from build123d import *

# Parameters (mm, degrees)
SKETCH1_W           = 241.3
SKETCH1_H           = 44.45
BOSS_EXTRUDE1_DEPTH = 19.06
SKETCH3_R           = 4
CUT_EXTRUDE1_DEPTH  = 125.151748779
CUT_EXTRUDE2_DEPTH  = 125.151748779
SKETCH11_R          = 15.113
CUT_EXTRUDE3_DEPTH  = 125.151748779
CUT_EXTRUDE5_DEPTH  = 125.151748779
FILLET1_R           = 3.175


with BuildPart() as part:
    # Sketch1 → Boss-Extrude1 (new body)
    with BuildSketch(Plane.XY):
        Rectangle(SKETCH1_W, SKETCH1_H)
    extrude(amount=BOSS_EXTRUDE1_DEPTH)

    # Sketch3 → Cut-Extrude1 (cut, through all)
    with BuildSketch(Plane.XY.offset(19.06)):
        with Locations((-107.95, 0)):
            Circle(SKETCH3_R)
    extrude(amount=-CUT_EXTRUDE1_DEPTH, mode=Mode.SUBTRACT)

    # Sketch5 → Cut-Extrude2 (cut, through all)
    with BuildSketch(Plane.XY.offset(19.06)):
        with BuildLine():
            ThreePointArc((67.637087091, -22.225), (96.497916739, -2.807923084), (120.65, 22.225))
            Line((120.65, 22.225), (120.65, -22.225))
            Line((120.65, -22.225), (67.637087091, -22.225))
        make_face()
        with BuildLine():
            Line((-61.710210997, -22.225), (-110.410681995, -9.201666649))
            ThreePointArc((-110.410681995, -9.201666649), (-117.466687359, 0.397852617), (-109.634072253, 9.374941368))
            Line((-109.634072253, 9.374941368), (-38.1, 22.225))
            Line((-38.1, 22.225), (-120.65, 22.225))
            Line((-120.65, 22.225), (-120.65, -22.225))
            Line((-120.65, -22.225), (-61.710210997, -22.225))
        make_face()
    extrude(amount=-CUT_EXTRUDE2_DEPTH, mode=Mode.SUBTRACT)

    # Sketch11 → Cut-Extrude3 (cut, through all)
    with BuildSketch(Plane(origin=(0, 0, 0), x_dir=(-1, 0, 0), z_dir=(0, 0, -1))):
        with Locations((-57.15, 0)):
            Circle(SKETCH11_R)
    extrude(amount=-CUT_EXTRUDE3_DEPTH, mode=Mode.SUBTRACT)

    # Sketch14 → Cut-Extrude5 (cut, through all)
    with BuildSketch(Plane.XY.offset(19.06)):
        Polygon((87.427282936, 15.558708401), (94.741989073, 6.41532573), (108.43714596, 17.350301349), align=None)
        Polygon((18.258483502, 14.338005817), (29.973493873, -13.800738505), (-32.606529101, -13.800738505), align=None)
        Polygon((-43.100879601, -13.800738505), (3.468328331, 11.961548148), (-56.519992491, 10.456326363), align=None)
        Polygon((-64.730780564, 8.662121496), (-52.068091334, -13.800738505), (-97.910045601, -2.558530136), align=None)
        Polygon((25.377220315, 10.456326363), (27.958556135, 4.256114298), (42.851089432, 10.456326363), align=None)
    extrude(amount=-CUT_EXTRUDE5_DEPTH, mode=Mode.SUBTRACT)

    # Fillet1
    # the kernel refuses this fillet: 3.175 mm, written as the material it adds along each edge
    with BuildSketch(Plane(origin=(-64.730780564, 8.662121496, 19.06), x_dir=(-0.9472961687281491, -0.32035912459764615, 0), z_dir=(0, 0, -1))) as fillet1_piece_1:
        with BuildLine():
            CenterArc((FILLET1_R * 0.828359701977, -FILLET1_R), FILLET1_R, 90, 79.273962625)
            Line((-FILLET1_R * 0.154168619156, -FILLET1_R * 0.813886867277), (0, 0))
            Line((0, 0), (FILLET1_R * 0.828359701977, 0))
        make_face()
    extrude(amount=19.06)
    with BuildSketch(Plane(origin=(-52.068091334, -13.800738505, 19.06), x_dir=(-0.9712208651423397, 0.23818066905642277, 0), z_dir=(0, 0, -1))) as fillet1_piece_2:
        with BuildLine():
            CenterArc((FILLET1_R * 2.310303232, FILLET1_R), FILLET1_R, 136.810131201, 133.189868799)
            Line((FILLET1_R * 1.58121357242, FILLET1_R * 1.68441819694), (0, 0))
            Line((0, 0), (FILLET1_R * 2.310303232, 0))
        make_face()
    extrude(amount=19.06)
    with BuildSketch(Plane(origin=(-97.910045601, -2.558530136, 19.06), x_dir=(0.9472961687281494, 0.32035912459764504, 0), z_dir=(0, 0, -1))) as fillet1_piece_3:
        with BuildLine():
            CenterArc((FILLET1_R * 3.43487976267, FILLET1_R), FILLET1_R, 122.463831423, 147.536168577)
            Line((FILLET1_R * 2.89811266126, FILLET1_R * 1.8437304539), (0, 0))
            Line((0, 0), (FILLET1_R * 3.43487976267, 0))
        make_face()
    extrude(amount=19.06)
    with BuildSketch(Plane(origin=(-56.519992491, 10.456326363, 19.06), x_dir=(0.9996853464994547, 0.025084018702456384, 0), z_dir=(0, 0, -1))) as fillet1_piece_4:
        with BuildLine():
            CenterArc((FILLET1_R * 1.64840949376, FILLET1_R), FILLET1_R, 152.485801408, 117.514198592)
            Line((FILLET1_R * 0.761513114746, FILLET1_R * 1.46196841114), (0, 0))
            Line((0, 0), (FILLET1_R * 1.64840949376, 0))
        make_face()
    extrude(amount=19.06)
    with BuildSketch(Plane(origin=(3.468328331, 11.961548148, 19.06), x_dir=(-0.8750292896969416, -0.48406997652453715, 0), z_dir=(0, 0, -1))) as fillet1_piece_5:
        with BuildLine():
            CenterArc((FILLET1_R * 4.08447056876, FILLET1_R), FILLET1_R, 117.514198592, 152.485801408)
            Line((FILLET1_R * 3.62250215761, FILLET1_R * 1.88689637901), (0, 0))
            Line((0, 0), (FILLET1_R * 4.08447056876, 0))
        make_face()
    extrude(amount=19.06)
    with BuildSketch(Plane(origin=(-43.100879601, -13.800738505, 19.06), x_dir=(0.8750292896969416, 0.48406997652453704, 0), z_dir=(0, 0, -1))) as fillet1_piece_6:
        with BuildLine():
            CenterArc((FILLET1_R, -FILLET1_R), FILLET1_R, 90, 90)
            Line((0, -FILLET1_R), (0, 0))
            Line((0, 0), (FILLET1_R, 0))
        make_face()
    extrude(amount=19.06)
    with BuildSketch(Plane(origin=(-32.606529101, -13.800738505, 19.06), x_dir=(0.8750292896969417, 0.48406997652453687, 0), z_dir=(0, 0, -1))) as fillet1_piece_7:
        with BuildLine():
            CenterArc((FILLET1_R * 3.87346743369, FILLET1_R), FILLET1_R, 118.951557757, 151.048442243)
            Line((FILLET1_R * 3.38939745717, FILLET1_R * 1.8750292897), (0, 0))
            Line((0, 0), (FILLET1_R * 3.87346743369, 0))
        make_face()
    extrude(amount=19.06)
    with BuildSketch(Plane(origin=(18.258483502, 14.338005817, 19.06), x_dir=(-0.8750292896969422, -0.4840699765245361, 0), z_dir=(0, 0, -1))) as fillet1_piece_8:
        with BuildLine():
            CenterArc((FILLET1_R * 1.11742055595, -FILLET1_R), FILLET1_R, 90, 96.348118808)
            Line((FILLET1_R * 0.123552109362, -FILLET1_R * 1.11056903214), (0, 0))
            Line((0, 0), (FILLET1_R * 1.11742055595, 0))
        make_face()
    extrude(amount=19.06)
    with BuildSketch(Plane(origin=(29.973493873, -13.800738505, 19.06), x_dir=(-1, 0, 0), z_dir=(0, 0, -1))) as fillet1_piece_9:
        with BuildLine():
            CenterArc((FILLET1_R * 1.49953423253, FILLET1_R), FILLET1_R, 157.396561051, 112.603438949)
            Line((FILLET1_R * 0.576347082868, FILLET1_R * 1.38435073396), (0, 0))
            Line((0, 0), (FILLET1_R * 1.49953423253, 0))
        make_face()
    extrude(amount=19.06)
    with BuildSketch(Plane(origin=(87.427282936, 15.558708401, 19.06), x_dir=(0.6246950475544248, -0.7808688094430298, 0), z_dir=(0, 0, -1))) as fillet1_piece_10:
        with BuildLine():
            CenterArc((FILLET1_R * 1.87227376636, -FILLET1_R), FILLET1_R, 90, 123.785764981)
            Line((FILLET1_R * 1.04115111223, -FILLET1_R * 1.55608914195), (0, 0))
            Line((0, 0), (FILLET1_R * 1.87227376636, 0))
        make_face()
    extrude(amount=19.06)
    with BuildSketch(Plane(origin=(108.43714596, 17.350301349, 19.06), x_dir=(-0.7814571605260681, -0.6239588978951538, 0), z_dir=(0, 0, -1))) as fillet1_piece_11:
        with BuildLine():
            CenterArc((FILLET1_R * 3.2984470476, FILLET1_R), FILLET1_R, 123.731770788, 146.268229212)
            Line((FILLET1_R * 2.74314138288, FILLET1_R * 1.83164633032), (0, 0))
            Line((0, 0), (FILLET1_R * 3.2984470476, 0))
        make_face()
    extrude(amount=19.06)
    with BuildSketch(Plane(origin=(94.741989073, 6.41532573, 19.06), x_dir=(-0.6246950475544234, 0.7808688094430309, 0), z_dir=(0, 0, -1))) as fillet1_piece_12:
        with BuildLine():
            CenterArc((FILLET1_R * 0.999058067303, FILLET1_R), FILLET1_R, 180.053994194, 89.946005806)
            Line((-FILLET1_R * 0.000941488660736, FILLET1_R * 0.999057623684), (0, 0))
            Line((0, 0), (FILLET1_R * 0.999058067303, 0))
        make_face()
    extrude(amount=19.06)
    with BuildSketch(Plane(origin=(27.958556135, 4.256114298, 19.06), x_dir=(-0.3843507339571626, 0.9231871496650018, 0), z_dir=(0, 0, -1))) as fillet1_piece_13:
        with BuildLine():
            CenterArc((FILLET1_R, FILLET1_R), FILLET1_R, 180, 90)
            Line((0, FILLET1_R), (0, 0))
            Line((0, 0), (FILLET1_R, 0))
        make_face()
    extrude(amount=19.06)
    with BuildSketch(Plane(origin=(42.851089432, 10.456326363, 19.06), x_dir=(-0.9231871496650015, -0.3843507339571632, 0), z_dir=(0, 0, -1))) as fillet1_piece_14:
        with BuildLine():
            CenterArc((FILLET1_R * 5.003729614, FILLET1_R), FILLET1_R, 112.603438949, 157.396561051)
            Line((FILLET1_R * 4.61937888005, FILLET1_R * 1.92318714967), (0, 0))
            Line((0, 0), (FILLET1_R * 5.003729614, 0))
        make_face()
    extrude(amount=19.06)
    with BuildSketch(Plane(origin=(25.377220315, 10.456326363, 19.06), x_dir=(0.3843507339571629, -0.9231871496650017, 0), z_dir=(0, 0, -1))) as fillet1_piece_15:
        with BuildLine():
            CenterArc((FILLET1_R * 1.49953423253, -FILLET1_R), FILLET1_R, 90, 112.603438949)
            Line((FILLET1_R * 0.576347082868, -FILLET1_R * 1.38435073396), (0, 0))
            Line((0, 0), (FILLET1_R * 1.49953423253, 0))
        make_face()
    extrude(amount=19.06)


solid = part.part
Geometry: final body of the model. Coordinates: model frame, mm. A direction names the side the tool comes from. Give positions to 0.01 mm unless a question says otherwise; leave off trailing zeros. Write each loop counter-clockwise with the first axis right and the second up, starting at its lowest first coordinate (ties: lowest second). Pieces come first, ordered by that corner, then holes. Notation, with made-up numbers: (14, -6) -> (33, -6) arc R21 cw to (33, 31) -> close; hole circle Ø1 at (82, -22). An arc over 180 degrees is marked (long way). Answer as a JSON object with one key per item and string values.
1. Mould query, pull axis X, two halves, no side actions, for faces 1 (the flat face through (40, 22.225, 9)), 2 (the flat face through (-49.38, -2.45, 9.66)), 3 (the cylindrical face through (-117.473, 0.218, 9.663)). Classes: pulls with the +X half, pulls with the -X half, needs draft (parallel to the pull), parting line crosses it, or undercut.
Ans:
{"face 1": "needs draft", "face 2": "undercut", "face 3": "pulls with the -X half"}
2. Cut plane A-A on x = -82.5. Output: boundary loops of the cut face in (y, z), and give its area (3 significant figures).
Ans:
{"outline": "(-16.67, 0) -> (-6.34, 0) -> (-6.34, 19.06) -> (-16.67, 19.06) -> close; (2.65, 0) -> (14.25, 0) -> (14.25, 19.06) -> (2.65, 19.06) -> close", "area": "418 mm^2"}
3. Cut plane B-B on z = 9.5. Count the separate pieces of the cut face and the enclosed holes in it, and give its area (3 significant figures).
Ans:
{"separate pieces": "1", "enclosed holes": "7", "area": "5,760 mm^2"}
4. Contact query for flat-ended pins moving along their axis: pin 1 (5 mm diameter, centred on y = -9, z = 5.5, fed in from -X); pin 2 (8 mm diameter, centred on x = 83, z = 7.5, fed in from -Y); pin 3 (3 mm diameter, centred on y = 8.5, z = 3.5, fed in from +X). Output: stop coordinate, or through.
Ans:
{"pin 1": "stops at x = -114.91", "pin 2": "stops at y = -15.62", "pin 3": "stops at x = 110.12"}
5. Ray query, probe 1 along Y at (x, z) = (57.15, 13) (3 decimals); probe 2 along X at (y, z) = (-2, 3.5); probe 3 along Y at (x, z) = (-12, 1) (3 decimals). Return the intervals inside material, ascending. Write a range as from..to.
Ans:
{"probe 1": "y = -22.225..-15.113, 15.113..22.225", "probe 2": "x = -117.26..-111.41, -104.49..-89.74, -58.72..-49.63, -21.77..-11.27, 25.06..42.17, 72.13..97.45", "probe 3": "y = -22.225..-13.801, -2.401..3.404, 11.573..22.225"}
6. Access query for faces 4 (the cylindrical face through (101.2, 14.53, 9.66)), 5 (the flat face through (-74.37, 15.71, 9.66)). Directions: +Z, -Z, +X, -X, +Y, -Y. A direction counts if a zero-diameter tool reaches every point of the face in a straight line with its end or side. Return the directions, or none.
Ans:
{"face 4": "+Z, -Z", "face 5": "+Z, -Z, -X, +Y"}
7. Cut plane C-C on x = 104. Output: boundary loops of the cut face in (y, z) (3 decimals), and give its area (3 significant figures).
Ans:
{"outline": "(3.882, 0) -> (22.225, 0) -> (22.225, 19.06) -> (3.882, 19.06) -> close", "area": "350 mm^2"}
